Autodesk Inventor part; units mm, degrees
ref_plane "YZ Plane" through (0, 0, 0) normal (1, 0, 0) x (0, 1, 0)
ref_plane "XZ Plane" through (0, 0, 0) normal (0, 1, 0) x (-1, 0, 0)
ref_plane "XY Plane" through (0, 0, 0) normal (0, 0, 1) x (1, 0, 0)
sketch "Sketch1" plane through (0, 0, 0) normal (0, 1, 0) x (-1, 0, 0)
  line L0 (0, 0) -> (-6.5, 0)
  line L1 (-6.5, 0) -> (-6.5, 8)
  line L2 (-6.5, 8) -> (-4, 8)
  line L3 (-4, 8) -> (-4, 23)
  line L4 (-4, 23) -> (0, 23)
  line L5 (0, 23) -> (0, 0)
  dimension "ScrewLength" = 15
  dimension "Diameter" = 13
  dimension "Metric" = 8
  dimension "HeadLength" = 8
revolve "Revolution1" add sketch "Sketch1" angle 360 about axis through (0, 0, 23) along (0, 0, -1)
thread "Thread1"
sketch "Sketch2" plane through (0, 0, 0) normal (0, 0, -1) x (-1, 0, 0)
  line L0 (1.7321, 3) -> (3.4641, 0)
  line L1 (3.4641, 0) -> (1.7321, -3)
  line L2 (1.7321, -3) -> (-1.7321, -3)
  line L3 (-1.7321, -3) -> (-3.4641, 0)
  line L4 (-3.4641, 0) -> (-1.7321, 3)
  line L5 (-1.7321, 3) -> (1.7321, 3)
  point P0 (0, 0)
  point P1 (0, 0)
  dimension "WidthAcrossFlat" = 6
extrude "Extrusion1" cut sketch "Sketch2" against normal blind 4
properties part number "UC-0815" material "Stainless Steel AISI 304"
Here's how the part is built. I have some questions about the finished solid (model axes, mm). A direction names the side the tool comes from. Give positions to 0.01 mm unless a question says otherwise; leave off trailing zeros. Order: outer loops, then holes, each group sorted by start corner. A loop starts at its lowest first (then second) coordinate and runs counter-clockwise, first axis right, second up. Notation, with made-up numbers: (20.25, 41.5) -> (44.25, 41.5) arc R14 cw to (44.25, 49.5) -> close; hole circle Ø9 at (27.25, 27.5). An arc over 180 degrees is marked (long way). One line per item, written item: value. Start each with the question number.
1. Imagine slicing it at A-A, the plane x = 0. List the corners of the cut face in (y, z) for me.
2. I need wall thicknesses on probe 1 along Z at (x, y) = (0, -5.75); probe 2 along Y at (x, z) = (5.5, 3.5); probe 3 along Y at (x, z) = (1, 1). Which ranges of each line are inside material? Lowest first, please. Write a range as from..to.
3. We'd pull the mould along Y, two halves only. Please class faces 4 (the face through (0, 0, 23)), 5 (the face through (-0.867, -3.905, 15.605)), 6 (the face through (0, 0, 4)): released by +Y, released by -Y, zero draft, split by the parting line, or undercut.
4. Will these pins go through, and if not, where does the flat tip stop? pin 1 Ø2 at (y, z) = (-3.5, 20) entering from +X; pin 2 Ø3 at (x, y) = (-0.5, 1) entering from -Z; pin 3 Ø5 at (x, y) = (5, 4) entering from +Z; pin 4 Ø3 at (y, z) = (2, 8) entering from +X.
5. Imagine slicing it at C-C, the plane z = 12.5. List the corners of the cut face in (x, y) for me, plus the area to 3 significant figures.
6. For faces 1 (the face through (3, -3, 8)), 2 (the face through (0, -3, 2)), 3 (the face through (-5.158, -3.955, 4.056)), which set-ups out of +Z, -Z, +X, -X, +Y, -Y let a thin tool reach every point of the face, with its end or its side?
7. Imagine slicing it at D-D, the plane z = 4.75. List the corners of the cut face in (x, y) for me.
8. Imagine slicing it at B-B, the plane y = -2. List the corners of the cut face in (x, z) for me, plus the area to 3 significant figures.
Values follow:
1. outline: (-6.5, 0) -> (-3, 0) -> (-3, 4) -> (3, 4) -> (3, 0) -> (6.5, 0) -> (6.5, 8) -> (4, 8) -> (4, 23) -> (-4, 23) -> (-4, 8) -> (-6.5, 8) -> close
2. probe 1: z = 0..8
2. probe 2: y = -3.46..3.46
2. probe 3: y = -6.42..-3, 3..6.42
3. face 4: zero draft
3. face 5: split by the parting line
3. face 6: undercut
4. pin 1: stops at x = 3.12
4. pin 2: stops at z = 4
4. pin 3: stops at z = 23
4. pin 4: stops at x = 6.48
5. outline: circle Ø8 at (0, 0)
5. area: 50.3 mm2
6. face 1: +Z
6. face 2: -Z
6. face 3: +Z, -Z
7. outline: circle Ø13 at (0, 0)
8. outline: (-6.18, 0) -> (-2.31, 0) -> (-2.31, 4) -> (2.31, 4) -> (2.31, 0) -> (6.18, 0) -> (6.18, 8) -> (3.46, 8) -> (3.46, 23) -> (-3.46, 23) -> (-3.46, 8) -> (-6.18, 8) -> close
8. area: 184 mm2
